Model file for the job. Use its own axes, mm. A direction names the side the tool comes from. Give positions to 0.01 mm unless a question says otherwise; leave off trailing zeros. Loops run counter-clockwise (first coordinate to the right, second up) from the corner with the lowest first, then second, coordinate; pieces in that order, holes last. Notation, with made-up numbers: (24, -30.75) - (52, -30.75) arc R9 cw to (52, -25.75) - close; hole circle Ø1 at (60, 63). An arc over 180 degrees is marked (long way). Use a Markdown table: item, result.
from build123d import *

# Parameters (mm, degrees)
F0_W     = 5
F0_H     = 8
F0_R     = 1.5
F1_DEPTH = 0.5
F0_W_2   = 2
F2_DEPTH = 2
F4_W     = 18
F4_H     = 8
F5_DEPTH = 1
F6_DEPTH = 2


with BuildPart() as f1:
    # F0 (on Top) → F1 (new body)
    with BuildSketch(Plane.XY):
        with Locations((-3.5, 0)):
            Rectangle(F0_W, F0_H)
        with Locations((-3, 0)):
            Circle(F0_R, mode=Mode.SUBTRACT)
        with Locations((3.5, 0)):
            Rectangle(F0_W, F0_H)
        with Locations((3, 0)):
            Circle(F0_R, mode=Mode.SUBTRACT)
    extrude(amount=F1_DEPTH)

    # F0 (on Top) → F2 (join)
    with BuildSketch(Plane.XY):
        Rectangle(F0_W_2, F0_H)
    extrude(amount=F2_DEPTH)

    # F4 (on offset) → F5 (join)
    with BuildSketch(Plane.XY.offset(2)):
        Rectangle(F4_W, F4_H)
    extrude(amount=F5_DEPTH)

    # F0 (on Top) → F6 (join)
    with BuildSketch(Plane.XY):
        with Locations((-3.5, 0)):
            Rectangle(F0_W, F0_H)
        with Locations((-3, 0)):
            Circle(F0_R, mode=Mode.SUBTRACT)
        Rectangle(F0_W_2, F0_H)
        with Locations((3.5, 0)):
            Rectangle(F0_W, F0_H)
        with Locations((3, 0)):
            Circle(F0_R, mode=Mode.SUBTRACT)
    extrude(amount=-F6_DEPTH)


solid = f1.part
(1) Slice it at D-D, the plane y = -2.25. Write the cut outline in (x, z).
Computed:
| item | result |
|---|---|
| outline | (-9, 2) - (-1, 2) - (-1, 0.5) - (-6, 0.5) - (-6, -2) - (6, -2) - (6, 0.5) - (1, 0.5) - (1, 2) - (9, 2) - (9, 3) - (-9, 3) - close |
(2) 3-axis set-ups, long thin cutter, end or side, ignore diameter. For faces 1 (the flat face through (-5, 0, 2)), 2 (the flat face through (5, 0, 2)), 3 (the flat face through (-6, 0, -1)), 4 (the flat face through (9, -0.1, 2.5)), 5 (the flat face through (6, 0, -1)): which of +Z, -Z, +X, -X, +Y, -Y reach the whole face in a straight line?
Computed:
| item | result |
|---|---|
| face 1 | -X, +Y, -Y |
| face 2 | +X, +Y, -Y |
| face 3 | -Z, -X, +Y, -Y |
| face 4 | +Z, -Z, +X, +Y, -Y |
| face 5 | -Z, +X, +Y, -Y |
(3) Slice it at B-B, the plane x = -3. Write the cut outline in (y, z), plus the area to 3 significant figures.
Computed:
| item | result |
|---|---|
| outline | (-4, -2) - (-1.5, -2) - (-1.5, 0.5) - (-4, 0.5) - close; (-4, 2) - (4, 2) - (4, 3) - (-4, 3) - close; (1.5, -2) - (4, -2) - (4, 0.5) - (1.5, 0.5) - close |
| area | 20.5 mm² |
(4) Drill centre lines: probe 1 along Z at (x, y) = (-2.25, -2); probe 2 along Y at (x, z) = (-3, -1.5); probe 3 along X at (y, z) = (-1, -0.7). Where is each one in solid material? Low to high. Write a range as [from, to].
Computed:
| item | result |
|---|---|
| probe 1 | [-2, 0.5], [2, 3] |
| probe 2 | [-4, -1.5], [1.5, 4] |
| probe 3 | [-6, -4.12], [-1.88, 1.88], [4.12, 6] |
(5) Slice it at C-C, the plane z = -1.55. Write the cut outline in (x, y).
Computed:
| item | result |
|---|---|
| outline | (-6, -4) - (6, -4) - (6, 4) - (-6, 4) - close; hole circle Ø3 at (-3, 0); hole circle Ø3 at (3, 0) |
(6) Mould opens along X. For faces 6 (the cylindrical face through (-1.57, 0.45, -0.77)), 7 (the flat face through (0, -4, 1)), 8 (the cylindrical face through (4.386, -0.575, -0.768)), 9 (the flat face through (-1, 0, 1)) say: pulls with the +X half, pulls with the -X half, needs draft (parallel to the pull), parting line crosses it, or undercut.
Computed:
| item | result |
|---|---|
| face 6 | undercut |
| face 7 | needs draft |
| face 8 | undercut |
| face 9 | pulls with the -X half |
(7) Pin check, flat tips, straight feed: P1, Ø3, axis at y = 0.5, z = -0.5, coming from the +X side; P2, Ø2.5, axis at x = -3, y = 0, coming from the -Z side; P3, Ø2, axis at y = 0, z = 0, coming from the -X side. Stop position of each tip, or through.
Computed:
| item | result |
|---|---|
| P1 | x = 6 |
| P2 | z = 2 |
| P3 | x = -6 |
(8) Slice it at A-A, the plane y = 0.75. Write the cut outline in (x, z), plus the area to 3 significant figures.
Computed:
| item | result |
|---|---|
| outline | (-9, 2) - (-1, 2) - (-1, 0.5) - (-1.7, 0.5) - (-1.7, -2) - (1.7, -2) - (1.7, 0.5) - (1, 0.5) - (1, 2) - (9, 2) - (9, 3) - (-9, 3) - close; (-6, -2) - (-4.3, -2) - (-4.3, 0.5) - (-6, 0.5) - close; (4.3, -2) - (6, -2) - (6, 0.5) - (4.3, 0.5) - close |
| area | 38.0 mm² |
